```python
from build123d import *

# Parameters (mm, degrees)
SKETCH_1_R               = 30
EXTRUDE_1_DEPTH          = 12
SKETCH_2_R               = 15
CUT_EXTRUDE_1_DEPTH      = 12
SKETCH_3_R               = 3
CUT_EXTRUDE_2_DEPTH      = 12
PATTERN_CIRCULAR_1_COUNT = 6


with BuildPart() as part:
    # 草图1 → 凸台-拉伸1 (new body)
    with BuildSketch(Plane(origin=(0, 0, 0), x_dir=(1, 0, 0), z_dir=(0, 1, 0))):
        with Locations(Location((0, 0, 0), (0, 0, 270))):
            Circle(SKETCH_1_R)
    extrude(amount=EXTRUDE_1_DEPTH)

    # 草图2 → 切除-拉伸1 (cut)
    with BuildSketch(Plane(origin=(0, 0, 0), x_dir=(1, 0, 0), z_dir=(0, 1, 0))):
        with Locations(Location((0, 0, 0), (0, 0, 270))):
            Circle(SKETCH_2_R)
    extrude(amount=CUT_EXTRUDE_1_DEPTH, mode=Mode.SUBTRACT)

    # 草图3 → 切除-拉伸2 (cut)
    with BuildSketch(Plane(origin=(0, 0, 0), x_dir=(1, 0, 0), z_dir=(0, 1, 0))):
        with Locations(Location((22, 0, 0), (0, 0, 270))):
            Circle(SKETCH_3_R)
    cut_extrude_2 = extrude(amount=CUT_EXTRUDE_2_DEPTH, mode=Mode.SUBTRACT)

    # 阵列(圆周)1: 切除-拉伸2 ×6 about axis
    pattern_circular_1_axis = Axis((0, 0, 0), (0, 1, 0))
    for i in range(1, PATTERN_CIRCULAR_1_COUNT):
        add(cut_extrude_2.rotate(pattern_circular_1_axis, i * 360 / PATTERN_CIRCULAR_1_COUNT), mode=Mode.SUBTRACT)


solid = part.part
```
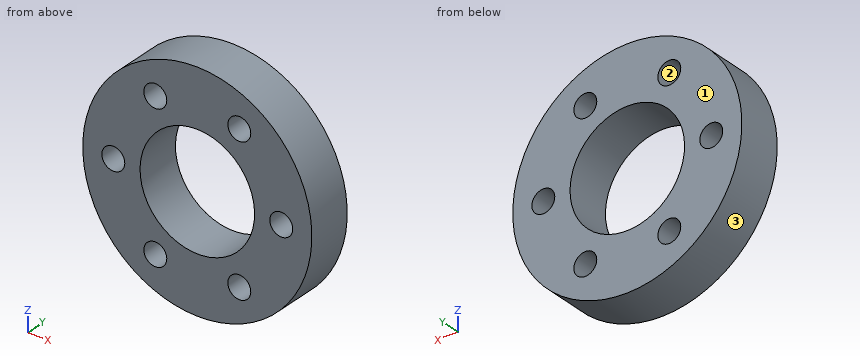
Geometry check sheet. Reference: the model listing, model coordinates, mm. Face numbers are marked on the shaded views. Coordinates: 2 decimals unless noted, no trailing zeros. Order: outer loops, then holes, each group sorted by start corner. A loop starts at its lowest first (then second) coordinate and runs counter-clockwise, first axis right, second up. Notation, with made-up numbers: M 48.25,88.5 L 103.25,88.5 A27 cw 103.25,124.5 Z; hole C -14,32.5 d1. An arc over 180 degrees is marked long. One line per question, with ' | ' between items. Start each with the question number.
Item 1: Cross-section at B-B on x = 0. Enter the section's corners in (y, z), then the cut area to 3 significant figures.
Item 2: Draft check along X on the marked faces 1, 2 and 3. Enter one of: pulls with the +X half, pulls with the -X half, needs draft (parallel to the pull), parting line crosses it, or undercut.
Item 3: Cross-section at C-C on z = 7. Enter the section's corners in (x, y), then the cut area to 3 significant figures.
Item 4: Cross-section at A-A on z = 0. Enter the section's corners in (x, y), then the cut area to 3 significant figures.
Item 5: Cross-section at D-D on x = 11. Enter the section's corners in (y, z), then the cut area to 3 significant figures.
Item 6: Material ranges on L1, parallel to X at y = 5, z = 0; L2, parallel to X at y = 4, z = -20.5; L3, parallel to X at y = 3.5, z = -20, recorded low to high. Write a range as [from, to].
Item 7: Gauge pin test, flat ends, axial feed: pin 1 (8 mm diameter, centred on x = -11, z = 19.05, fed in from -Y); pin 2 (1 mm diameter, centred on y = 7.5, z = 15, fed in from +X); pin 3 (1.5 mm diameter, centred on y = 10.5, z = -0.5, fed in from +X); pin 4 (6 mm diameter, centred on x = -18, y = 4, fed in from +Z). Record the tip position at first contact, or that the pin passes through.
Findings:
1) outline: M 0,-30 L 12,-30 L 12,-15 L 0,-15 Z; M 0,15 L 12,15 L 12,30 L 0,30 Z | area: 360 mm²
2) face 1: needs draft | face 2: undercut | face 3: parting line crosses it
3) outline: M -29.17,0 L -13.27,0 L -13.27,12 L -29.17,12 Z; M 13.27,0 L 29.17,0 L 29.17,12 L 13.27,12 Z | area: 382 mm²
4) outline: M -30,0 L -25,0 L -25,12 L -30,12 Z; M -19,0 L -15,0 L -15,12 L -19,12 Z; M 15,0 L 19,0 L 19,12 L 15,12 Z; M 25,0 L 30,0 L 30,12 L 25,12 Z | area: 216 mm²
5) outline: M 0,-27.91 L 12,-27.91 L 12,-22.05 L 0,-22.05 Z; M 0,-16.05 L 12,-16.05 L 12,-10.2 L 0,-10.2 Z; M 0,10.2 L 12,10.2 L 12,16.05 L 0,16.05 Z; M 0,22.05 L 12,22.05 L 12,27.91 L 0,27.91 Z | area: 281 mm²
6) L1: x = [-30, -25], [-19, -15], [15, 19], [25, 30] | L2: x = [-21.9, -13.63], [-8.37, 8.37], [13.63, 21.9] | L3: x = [-22.36, -13.85], [-8.15, 8.15], [13.85, 22.36]
7) pin 1: stops at y = 0 | pin 2: stops at x = 26.26 | pin 3: stops at x = 30 | pin 4: stops at z = 25.98
